Geometry check sheet. Reference: the model listing, model coordinates, mm. Face numbers are marked on the shaded views. A direction names the side the tool comes from. Round coordinates to 2 decimals unless told otherwise and drop trailing zeros. Loops run counter-clockwise (first coordinate to the right, second up) from the corner with the lowest first, then second, coordinate; pieces in that order, holes last. Notation, with made-up numbers: (38.5, 89) -> (60.5, 89) arc R22 cw to (60.5, 128) -> close; hole circle Ø2 at (-16.75, 2.5). An arc over 180 degrees is marked (long way). Use a Markdown table: item, result. Add a question column.
Q1. Material ranges on L1, parallel to Y at x = 29, z = -5; L2, parallel to Y at x = 3, z = 15; L3, parallel to X at y = 125, z = 29, recorded low to high.
Q2. Release check for a two-part mould opening along X. For the marked faces 1, 2 and 3 record: released by +X, released by -X, zero draft, split by the parting line, or undercut.
Q3. Gauge pin test, flat ends, axial feed: P1, Ø6, axis at y = 28, z = 20, coming from the +X side; P2, Ø1.5, axis at x = -37.5, z = 5.5, coming from the +Y side; P3, Ø10, axis at y = 107, z = 15, coming from the +X side. Record the tip position at first contact, or that the pin passes through.
Q4. Sectioned sample at A-A, the plane y = 146. Enter the section's corners in (x, z).
Q5. Set-up check for the marked faces 4, 5, 6 and 7: record each of +Z, -Z, +X, -X, +Y, -Y from which the full face is reachable in a straight line by a thin tool's end or side.
Q6. Sectioned sample at B-B, the plane y = 84. Enter the section's corners in (x, z), then the cut area to 3 significant figures.
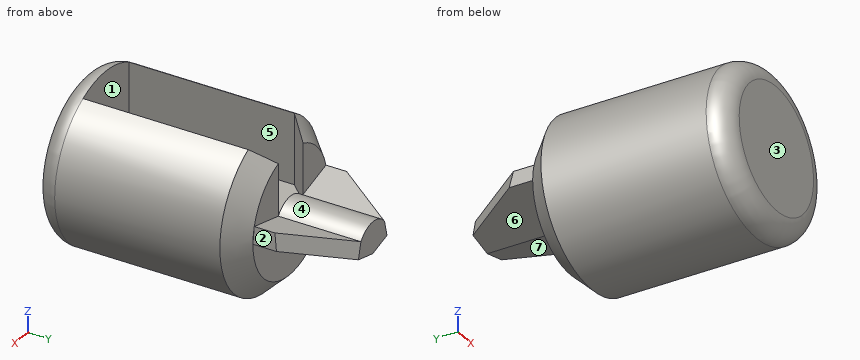
```python
from build123d import *

# Parameters (mm, degrees)
SKETCH1_R           = 50.8
BOSS_EXTRUDE1_DEPTH = 127
FILLET2_R           = 12.7
CHAMFER1_SIZE       = 12.7
BOSS_EXTRUDE2_DEPTH = 50.8
CUT_EXTRUDE2_DEPTH  = 193.012728369
CUT_EXTRUDE3_DEPTH  = 193.012728396
BOSS_EXTRUDE3_DEPTH = 50.8
CUT_EXTRUDE4_REACH  = 193.766


with BuildPart() as part:
    # Sketch1 → Boss-Extrude1 (new body)
    with BuildSketch(Plane(origin=(0, 0, 0), x_dir=(1, 0, 0), z_dir=(0, 1, 0))):
        with Locations(Location((0, 0, 0), (0, 0, 270))):
            Circle(SKETCH1_R)
    extrude(amount=BOSS_EXTRUDE1_DEPTH)

    # Fillet2
    fillet2_edges = [part.edges().sort_by_distance(p)[0] for p in [
        (0, 0, -50.8),
    ]]
    fillet(fillet2_edges, radius=FILLET2_R)

    # Chamfer1
    chamfer1_edges = [part.edges().sort_by_distance(p)[0] for p in [
        (0, 127, -50.8),
    ]]
    chamfer(chamfer1_edges, length=CHAMFER1_SIZE)

    # Sketch2 → Boss-Extrude2 (add)
    with BuildSketch(Plane(origin=(0, 127, 0), x_dir=(1, 0, 0), z_dir=(0, 1, 0))):
        Polygon((0, 9.725532547), (-38.1, -4.635e-06), (-36.720352746, -10.160004635), (0, -0.786640962), (36.720352746, -10.160004635), (38.1, -4.635e-06), align=None)
    extrude(amount=BOSS_EXTRUDE2_DEPTH)

    # Sketch3 → Cut-Extrude2 (cut, through all)
    with BuildSketch(Plane(origin=(0.18851702, 0, 0.738519458), x_dir=(0.9689306468108195, 0, -0.24733257300801867), z_dir=(0.2473325730080187, 0, 0.9689306468108196))):
        Polygon((-38.092375226, 139.7), (-38.092375226, 177.8), (-12.692375226, 177.8), align=None)
    extrude(amount=-CUT_EXTRUDE2_DEPTH, mode=Mode.SUBTRACT)

    # Sketch4 → Cut-Extrude3 (cut, through all)
    with BuildSketch(Plane(origin=(-0.18851702, 0, 0.738519458), x_dir=(0.9689306468108199, 0, 0.24733257300801748), z_dir=(-0.24733257300801748, 0, 0.9689306468108199))):
        Polygon((12.692375226, 177.8), (38.092375226, 177.8), (38.092375226, 139.7), align=None)
    extrude(amount=-CUT_EXTRUDE3_DEPTH, mode=Mode.SUBTRACT)

    # Sketch5 → Boss-Extrude3 (add)
    with BuildSketch(Plane(origin=(0, 127, 0), x_dir=(1, 0, 0), z_dir=(0, 1, 0))):
        with BuildLine():
            Line((-12.109514317, -3.87775728), (0, -0.786640962))
            Line((0, -0.786640962), (12.109514317, -3.87775728))
            ThreePointArc((12.109514317, -3.87775728), (0, -9.864797592), (-12.109514317, -3.87775728))
        make_face()
    extrude(amount=BOSS_EXTRUDE3_DEPTH)

    # Sketch6 → Cut-Extrude4 (cut, up to next)
    with BuildSketch(Plane.XY, mode=Mode.PRIVATE) as cut_extrude4_sk1:
        Polygon((-13.290485683, 127), (-25.4, 114.3), (-25.4, 12.7), (21.819967816, 12.7), (21.819967816, 114.3), (12.109514317, 127), align=None)
    cut_extrude4_tool1 = extrude(cut_extrude4_sk1.sketch, amount=CUT_EXTRUDE4_REACH, mode=Mode.PRIVATE) & part.part
    add(cut_extrude4_tool1.solids().sort_by_distance((-1.74269, 68.455742, 0))[0], mode=Mode.SUBTRACT)


solid = part.part
```
Values:
| question | item | result |
|---|---|---|
| 1 | L1 | 0 to 127 |
| 1 | L2 | 0 to 12.7 |
| 1 | L3 | -27.69 to -15.2, 13.64 to 27.69 |
| 2 | face 1 | undercut |
| 2 | face 2 | released by +X |
| 2 | face 3 | zero draft |
| 3 | P1 | x = 47.87 |
| 3 | P2 | y = 141.42 |
| 3 | P3 | x = 49.81 |
| 4 | outline | (-35.17, -0.75) -> (0, -9.73) -> (35.17, -0.75) -> (32.65, 9.12) -> (12.11, 3.88) arc R15.24 ccw to (-12.11, 3.88) -> (-32.65, 9.12) -> close |
| 5 | face 4 | +Z, +Y |
| 5 | face 5 | +Z |
| 5 | face 6 | -Z, -X, +Y |
| 5 | face 7 | -Z, +X, +Y |
| 6 | outline | (-25.4, 0) -> (-25.4, 43.99) arc R50.8 ccw (long way) to (21.82, 45.88) -> (21.82, 0) -> close |
| 6 | area | 5,800 mm^2 |
